Build history of the part. All positions in model axes, mm. A direction names the side the tool comes from. Give positions to 0.01 mm unless a question says otherwise; leave off trailing zeros. Loops run counter-clockwise (first coordinate to the right, second up) from the corner with the lowest first, then second, coordinate; pieces in that order, holes last. Notation, with made-up numbers: M 84,22.25 L 103,22.25 A24 ccw 103,54.25 Z; hole C 77,17 d6. An arc over 180 degrees is marked long. Answer in a Markdown table with one row per item. Add a question column.
```python
from build123d import *

# Parameters (mm, degrees)
F1_DEPTH = 76.2
F3_DEPTH = 152.4


with BuildPart() as f1:
    # F0 (on Front) → F1 (new body)
    with BuildSketch(Plane.XZ):
        Polygon((-76.556332, 50.8), (-76.556332, 0), (75.843668, 0), (75.843668, 38.1), (39.717197, 38.1), (10.648812, 38.1), (1.046149, 50.8), (-24.353851, 50.8), (-24.353851, 38.1), (-11.653851, 38.1), (-11.653851, 25.4), (-62.453851, 25.4), (-62.453851, 38.1), (-51.156332, 38.1), (-51.156332, 50.8), align=None)
    extrude(amount=F1_DEPTH)

    # F2 (on face) → F3 (cut, through all)
    with BuildSketch(Plane.YZ.offset(75.843668)):
        Polygon((-62.453851, 10.936619), (-50.8, 0), (-27.053742, 0), (-15.253706, 10.936619), align=None)
    extrude(amount=-F3_DEPTH, mode=Mode.SUBTRACT)


solid = f1.part
```
(1) Slice it at B-B, the plane x = -59.5. Give the cut face in (y, z).
(2) Pull direction Z, two halves, no side cores. Call faces 1 (the flat face through (-1, -13, 0)), 2 (the flat face through (-11.654, -38, 32)), 3 (the flat face through (-24.354, -38, 45)), 4 (the flat face through (5.915, -37.567, 44.361)): +Z half, -Z half, draft (parallel to the pull), parting line (faces both ways), or undercut.
(3) Slice it at A-A, the plane z = 34. Give the cut face in (x, y).
(4) Wall check: line 1 (X direction, y = -5, z = 29.5); line 2 (Z direction, x = -23.5, y = -36); line 3 (Z direction, x = -54.5, y = -57.5). Give the ranges that are in metal, low to high.
(5) Tool access for faces 5 (the flat face through (-51.156, -38, 44)), 6 (the flat face through (0.71, -21.24, 5.39)), 7 (the flat face through (-37, -38, 25.4)), 8 (the flat face through (44, -38, 38.1)): list every direction of +Z, -Z, +X, -X, +Y, -Y with a clear straight run to the whole face (end or side of a thin tool).
(6) Slice it at D-D, the plane x = -9. Give the cut face in (y, z).
(7) Pin check, flat tips, straight feed: pin 1 (14 mm diameter, centred on x = -21, y = -19.5, fed in from -Z); pin 2 (8 mm diameter, centred on x = -39.5, y = -44, fed in from -Z); pin 3 (5 mm diameter, centred on x = 52.5, y = -60.5, fed in from +Z). Stop position of each tip, or through.
(8) Slice it at C-C, the plane y = -69.5. Give the cut face in (x, z).
Solution:
| question | item | result |
|---|---|---|
| 1 | outline | M -76.2,0 L -50.8,0 L -62.45,10.94 L -15.25,10.94 L -27.05,0 L 0,0 L 0,25.4 L -76.2,25.4 Z; M -76.2,38.1 L 0,38.1 L 0,50.8 L -76.2,50.8 Z |
| 2 | face 1 | -Z half |
| 2 | face 2 | undercut |
| 2 | face 3 | draft |
| 2 | face 4 | +Z half |
| 3 | outline | M -76.56,-76.2 L -62.45,-76.2 L -62.45,0 L -76.56,0 Z; M -11.65,-76.2 L 75.84,-76.2 L 75.84,0 L -11.65,0 Z |
| 4 | line 1 | -76.56 to -62.45, -11.65 to 75.84 |
| 4 | line 2 | 10.94 to 25.4, 38.1 to 50.8 |
| 4 | line 3 | 0 to 6.29, 10.94 to 25.4, 38.1 to 50.8 |
| 5 | face 5 | +Z, +Y, -Y |
| 5 | face 6 | +X, -X |
| 5 | face 7 | +Y, -Y |
| 5 | face 8 | +Z, +X, +Y, -Y |
| 6 | outline | M -76.2,0 L -50.8,0 L -62.45,10.94 L -15.25,10.94 L -27.05,0 L 0,0 L 0,50.8 L -76.2,50.8 Z |
| 7 | pin 1 | z = 0 |
| 7 | pin 2 | z = 10.94 |
| 7 | pin 3 | z = 38.1 |
| 8 | outline | M -76.56,0 L 75.84,0 L 75.84,38.1 L 10.65,38.1 L 1.05,50.8 L -24.35,50.8 L -24.35,38.1 L -11.65,38.1 L -11.65,25.4 L -62.45,25.4 L -62.45,38.1 L -51.16,38.1 L -51.16,50.8 L -76.56,50.8 Z |
